The drawing under review shows one solid part. Ordinate dimensions are in mm from its lowest x, y, z. A direction names the side the tool comes from. Give positions to 0.01 mm unless a question says otherwise; leave off trailing zeros. Loops run counter-clockwise (first coordinate to the right, second up) from the corner with the lowest first, then second, coordinate; pieces in that order, holes last.
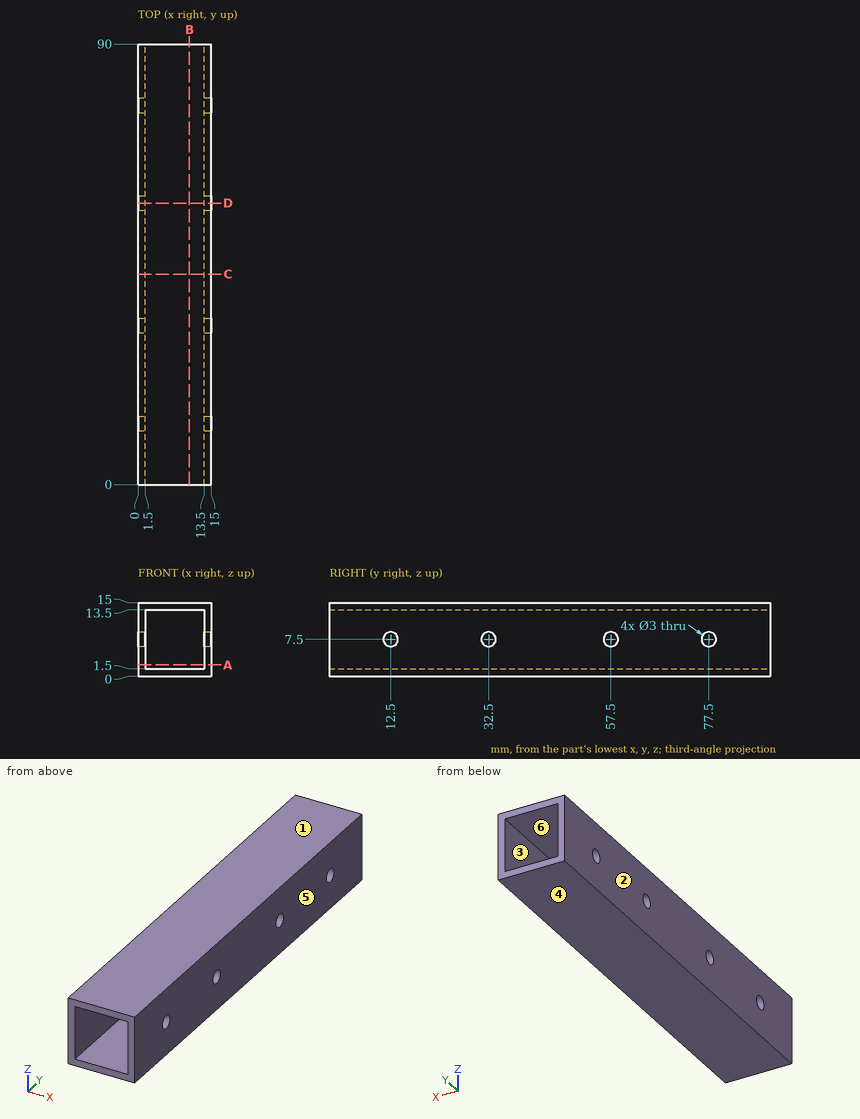
Item 1: Take a section at B-B on x = 10.5. Give the boundary of the cut face in (y, z).
Answer:
outline: (0, 0) - (90, 0) - (90, 1.5) - (0, 1.5) - close; (0, 13.5) - (90, 13.5) - (90, 15) - (0, 15) - close
Item 2: Take a section at A-A on z = 2.25. Give the boundary of the cut face in (x, y), and give its area (3 significant figures).
Answer:
outline: (0, 0) - (1.5, 0) - (1.5, 90) - (0, 90) - close; (13.5, 0) - (15, 0) - (15, 90) - (13.5, 90) - close
area: 270 mm2
Item 3: Tool access review of the marked faces 5 and 6: name each direction out of +Z, -Z, +X, -X, +Y, -Y from which nothing blocks a thin tool from reaching the whole face with its end or side.
Answer:
face 5: +Z, -Z, +X, +Y, -Y
face 6: +Y, -Y
Item 4: For L1, parallel to Y at x = 1.1, z = 7.5; L2, parallel to X at y = 20, z = 2.5, list the stretches that pass through material, from the lowest coordinate up.
Answer:
L1: y = 0 to 11, 14 to 31, 34 to 56, 59 to 76, 79 to 90
L2: x = 0 to 1.5, 13.5 to 15
Item 5: Take a section at C-C on y = 43. Give the boundary of the cut face in (x, z), and give its area (3 significant figures).
Answer:
outline: (0, 0) - (15, 0) - (15, 15) - (0, 15) - close; hole (1.5, 1.5) - (13.5, 1.5) - (13.5, 13.5) - (1.5, 13.5) - close
area: 81.0 mm2
Item 6: Take a section at D-D on y = 57.5. Give the boundary of the cut face in (x, z).
Answer:
outline: (0, 0) - (15, 0) - (15, 6) - (13.5, 6) - (13.5, 1.5) - (1.5, 1.5) - (1.5, 6) - (0, 6) - close; (0, 9) - (1.5, 9) - (1.5, 13.5) - (13.5, 13.5) - (13.5, 9) - (15, 9) - (15, 15) - (0, 15) - close
Item 7: Clearance check with a flat-ended pin moving along its axis: pin 1 Ø1.8 at (y, z) = (12.5, 7.5) entering from -X. State where the tip first meets the part, or that it passes through.
Answer:
pin 1: passes through
Item 8: The part is to be moulded in two halves that separate along Z. For the marked faces 1, 2, 3 and 4, say which applies: released by +Z, released by -Z, zero draft, split by the parting line, or undercut.
Answer:
face 1: released by +Z
face 2: zero draft
face 3: undercut
face 4: released by -Z
